Input: part model. Units: mm. Frame: model coordinates. Face numbers are marked on the shaded views. A direction names the side the tool comes from. Round coordinates to 2 decimals unless told otherwise and drop trailing zeros. Loops run counter-clockwise (first coordinate to the right, second up) from the corner with the lowest first, then second, coordinate; pieces in that order, holes last.
(1) Cut plane A-A, the plane y = 19. Output: boundary loops of the cut face in (x, z).
(2) First-contact query: pin 1 Ø2 at (y, z) = (48.5, 7.5) entering from +X; pin 2 Ø1.2 at (x, z) = (141, 14) entering from -Y; pin 3 Ø4.5 at (x, y) = (135.5, 22.5) entering from +Z; pin 4 Ø3 at (x, z) = (141.5, 14) entering from -Y. Flat tips, straight axial feed; report the tip coordinate or a pass-through.
(3) Cut plane B-B, the plane x = 141.5. Give the number of separate pieces and of enclosed holes in the cut face, and give its area (3 significant figures).
(4) Draft query along Y for the marked faces 5, 6 and 7. Return one class per face: released by +Y, released by -Y, zero draft, split by the parting line, or undercut.
(5) Cut plane C-C, the plane y = 31. Output: boundary loops of the cut face in (x, z).
(6) Cut plane D-D, the plane x = 147.5. Output: boundary loops of the cut face in (y, z).
(7) Line query: line 1 (Y direction, x = 133, z = 14); line 2 (Z direction, x = 141.5, y = 65); line 3 (Y direction, x = 136.75, z = 14). Output: solid intervals per line, ascending.
(8) Access query for the marked faces 1, 2, 3 and 4. Directions: +Z, -Z, +X, -X, +Y, -Y. A direction counts if a zero-diameter tool reaches every point of the face in a straight line with its end or side. Return the directions, or none.
from build123d import *

# Parameters (mm, degrees)
CYLINDER357_R     = 3
CYLINDER357_DEPTH = 17
CYLINDER356_R     = 3
CYLINDER356_DEPTH = 17
BOX221_W          = 5
BOX221_H          = 8
BOX221_DEPTH      = 10
FILLET089_R       = 2
BOX222_W          = 5
BOX222_H          = 60
BOX222_DEPTH      = 10
BOX217_W          = 1
BOX217_H          = 32
BOX217_DEPTH      = 22
CYLINDER297_R     = 1.6
CYLINDER297_DEPTH = 16
CYLINDER296_R     = 1.6
CYLINDER296_DEPTH = 16
CYLINDER295_R     = 1.25
CYLINDER295_DEPTH = 10
CYLINDER293_R     = 1.25
CYLINDER293_DEPTH = 10
CYLINDER294_R     = 1.25
CYLINDER294_DEPTH = 10
CYLINDER292_R     = 1.25
CYLINDER292_DEPTH = 10
CYLINDER291_R     = 3.5
CYLINDER291_DEPTH = 4
CYLINDER289_R     = 6.5
CYLINDER289_DEPTH = 4
BOX218_W          = 15
BOX218_H          = 16
BOX218_DEPTH      = 5.5
CYLINDER290_R     = 8
CYLINDER290_DEPTH = 10
BOX216_W          = 10
BOX216_H          = 80
BOX216_DEPTH      = 10
BOX219_W          = 5
BOX219_H          = 80
BOX219_DEPTH      = 10
FILLET090_R       = 2
BOX220_W          = 5
BOX220_H          = 8
BOX220_DEPTH      = 10
FILLET088_R       = 2
CHAMFER031_SIZE   = 5.49
CHAMFER032_SIZE   = 3
FILLET110_R       = 4.99


with BuildPart() as cylinder357:
    # Cylinder357 → Cylinder357 (new body)
    with BuildSketch(Plane(origin=(129, 57, 19), x_dir=(0, 0, -1), z_dir=(1, 0, 0))):
        Circle(CYLINDER357_R)
    extrude(amount=CYLINDER357_DEPTH)


with BuildPart() as fusion302:
    # Cylinder356 → Cylinder356 (new body)
    with BuildSketch(Plane(origin=(129, 5, 19), x_dir=(0, 0, -1), z_dir=(1, 0, 0))):
        Circle(CYLINDER356_R)
    extrude(amount=CYLINDER356_DEPTH)

    # Fusion302: union Cylinder357
    add(cylinder357.part)


with BuildPart() as fillet089:
    # Box221 → Box221 (new body)
    with BuildSketch(Plane(origin=(90, 53, 9), x_dir=(1, 0, 0), z_dir=(0, 0, 1))):
        with Locations((2.5, 4)):
            Rectangle(BOX221_W, BOX221_H)
    extrude(amount=BOX221_DEPTH)

    # Fillet089
    fillet089_edges = [fillet089.edges().sort_by_distance(p)[0] for p in [
        (92.5, 61, 19),
    ]]
    fillet(fillet089_edges, radius=FILLET089_R)


with BuildPart() as fillet089_1:
    # Fillet089 placement: moved
    add(fillet089.part.moved(Location((0, 10, 0))))


with BuildPart() as cube302:
    # Box222 → Box222 (new body)
    with BuildSketch(Plane(origin=(75, 1, -1), x_dir=(1, 0, 0), z_dir=(0, 0, 1))):
        with Locations((2.5, 30)):
            Rectangle(BOX222_W, BOX222_H)
    extrude(amount=BOX222_DEPTH)


with BuildPart() as cube297:
    # Box217 → Box217 (new body)
    with BuildSketch(Plane(origin=(89, 15, 2), x_dir=(1, 0, 0), z_dir=(0, 0, 1))):
        with Locations((0.5, 16)):
            Rectangle(BOX217_W, BOX217_H)
    extrude(amount=BOX217_DEPTH)


with BuildPart() as cylinder297:
    # Cylinder297 → Cylinder297 (new body)
    with BuildSketch(Plane(origin=(80, 43, 14), x_dir=(0, 0, -1), z_dir=(1, 0, 0))):
        Circle(CYLINDER297_R)
    extrude(amount=CYLINDER297_DEPTH)


with BuildPart() as fusion262:
    # Cylinder296 → Cylinder296 (new body)
    with BuildSketch(Plane(origin=(80, 19, 14), x_dir=(0, 0, -1), z_dir=(1, 0, 0))):
        Circle(CYLINDER296_R)
    extrude(amount=CYLINDER296_DEPTH)

    # Fusion262: union Cylinder297
    add(cylinder297.part)


with BuildPart() as fusion262_1:
    # Fusion262 placement: moved
    add(fusion262.part.moved(Location((-6, 0, 0))))


with BuildPart() as cylinder295:
    # Cylinder295 → Cylinder295 (new body)
    with BuildSketch(Plane(origin=(87.5, 71, 14), x_dir=(1, 0, 0), z_dir=(0, -1, 0))):
        Circle(CYLINDER295_R)
    extrude(amount=CYLINDER295_DEPTH)


with BuildPart() as fusion260:
    # Cylinder293 → Cylinder293 (new body)
    with BuildSketch(Plane(origin=(87.5, 1, 14), x_dir=(1, 0, 0), z_dir=(0, -1, 0))):
        Circle(CYLINDER293_R)
    extrude(amount=CYLINDER293_DEPTH)

    # Fusion260: union Cylinder295
    add(cylinder295.part)


with BuildPart() as cylinder294:
    # Cylinder294 → Cylinder294 (new body)
    with BuildSketch(Plane(origin=(82.5, 71, 14), x_dir=(1, 0, 0), z_dir=(0, -1, 0))):
        Circle(CYLINDER294_R)
    extrude(amount=CYLINDER294_DEPTH)


with BuildPart() as fusion261:
    # Cylinder292 → Cylinder292 (new body)
    with BuildSketch(Plane(origin=(82.5, 1, 14), x_dir=(1, 0, 0), z_dir=(0, -1, 0))):
        Circle(CYLINDER292_R)
    extrude(amount=CYLINDER292_DEPTH)

    # Fusion259: union Cylinder294
    add(cylinder294.part)

    # Fusion261: union Fusion260
    add(fusion260.part)


with BuildPart() as cylinder291:
    # Cylinder291 → Cylinder291 (new body)
    with BuildSketch(Plane(origin=(89.5, 31, 10), x_dir=(0, 0, -1), z_dir=(1, 0, 0))):
        Circle(CYLINDER291_R)
    extrude(amount=CYLINDER291_DEPTH)


with BuildPart() as fusion257:
    # Cylinder289 → Cylinder289 (new body)
    with BuildSketch(Plane(origin=(90, 31, 10), x_dir=(0, 0, -1), z_dir=(1, 0, 0))):
        Circle(CYLINDER289_R)
    extrude(amount=CYLINDER289_DEPTH)

    # Fusion257: union Cylinder291
    add(cylinder291.part)


with BuildPart() as fusion257_1:
    # Fusion257 placement: moved
    add(fusion257.part.moved(Location((-4, 0, 2))))


with BuildPart() as cube298:
    # Box218 → Box218 (new body)
    with BuildSketch(Plane(origin=(75, 23, 3.5), x_dir=(1, 0, 0), z_dir=(0, 0, 1))):
        with Locations((7.5, 8)):
            Rectangle(BOX218_W, BOX218_H)
    extrude(amount=BOX218_DEPTH)


with BuildPart() as cylinder290:
    # Cylinder290 → Cylinder290 (new body)
    with BuildSketch(Plane(origin=(80, 31, 11.5), x_dir=(0, 0, -1), z_dir=(1, 0, 0))):
        Circle(CYLINDER290_R)
    extrude(amount=CYLINDER290_DEPTH)


with BuildPart() as fusion258:
    # Box216 → Box216 (new body)
    with BuildSketch(Plane(origin=(80, -9, 9), x_dir=(1, 0, 0), z_dir=(0, 0, 1))):
        with Locations((5, 40)):
            Rectangle(BOX216_W, BOX216_H)
    extrude(amount=BOX216_DEPTH)

    # Fusion258: union Cylinder290
    add(cylinder290.part)


with BuildPart() as fillet090:
    # Box219 → Box219 (new body)
    with BuildSketch(Plane(origin=(75, -9, 9), x_dir=(1, 0, 0), z_dir=(0, 0, 1))):
        with Locations((2.5, 40)):
            Rectangle(BOX219_W, BOX219_H)
    extrude(amount=BOX219_DEPTH)

    # Fusion263: union Cube298, Fusion258
    add(cube298.part)
    add(fusion258.part)

    # Cut226: cut Fusion257
    add(fusion257_1.part, mode=Mode.SUBTRACT)

    # Cut227: cut Fusion261
    add(fusion261.part, mode=Mode.SUBTRACT)

    # Cut228: cut Fusion262
    add(fusion262_1.part, mode=Mode.SUBTRACT)

    # Cut229: cut Cube297
    add(cube297.part, mode=Mode.SUBTRACT)

    # Cut230: cut Cube302
    add(cube302.part, mode=Mode.SUBTRACT)

    # Fillet090
    fillet090_edges = [fillet090.edges().sort_by_distance(p)[0] for p in [
        (82.5, -9, 19),
        (82.5, 71, 19),
    ]]
    fillet(fillet090_edges, radius=FILLET090_R)


with BuildPart() as front_threaded_bar_support_wide:
    # Box220 → Box220 (new body)
    with BuildSketch(Plane(origin=(90, 1, 9), x_dir=(1, 0, 0), z_dir=(0, 0, 1))):
        with Locations((2.5, 4)):
            Rectangle(BOX220_W, BOX220_H)
    extrude(amount=BOX220_DEPTH)

    # Fillet088
    fillet088_edges = [front_threaded_bar_support_wide.edges().sort_by_distance(p)[0] for p in [
        (92.5, 1, 19),
    ]]
    fillet(fillet088_edges, radius=FILLET088_R)


with BuildPart() as front_threaded_bar_support_wide_1:
    # Fillet088 placement: moved
    add(front_threaded_bar_support_wide.part.moved(Location((0, -10, 0))))

    # Fusion264: union Fillet089, Fillet090
    add(fillet089_1.part)
    add(fillet090.part)


with BuildPart() as front_threaded_bar_support_wide_2:
    # Fusion264 placement: moved
    add(front_threaded_bar_support_wide_1.part.moved(Location((54, 0, 0))))

    # Cut305: cut Fusion302
    add(fusion302.part, mode=Mode.SUBTRACT)

    # Chamfer031
    chamfer031_edges = [front_threaded_bar_support_wide_2.edges().sort_by_distance(p)[0] for p in [
        (138.5, 39, 9),
        (138.5, 23, 9),
    ]]
    chamfer(chamfer031_edges, length=CHAMFER031_SIZE)

    # Chamfer032
    chamfer032_edges = [front_threaded_bar_support_wide_2.edges().sort_by_distance(p)[0] for p in [
        (134, 31, 3.5),
    ]]
    chamfer(chamfer032_edges, length=CHAMFER032_SIZE)

    # Fillet110
    fillet110_edges = [front_threaded_bar_support_wide_2.edges().sort_by_distance(p)[0] for p in [
        (144, 63, 14),
        (144, -1, 14),
    ]]
    fillet(fillet110_edges, radius=FILLET110_R)


solid = front_threaded_bar_support_wide_2.part
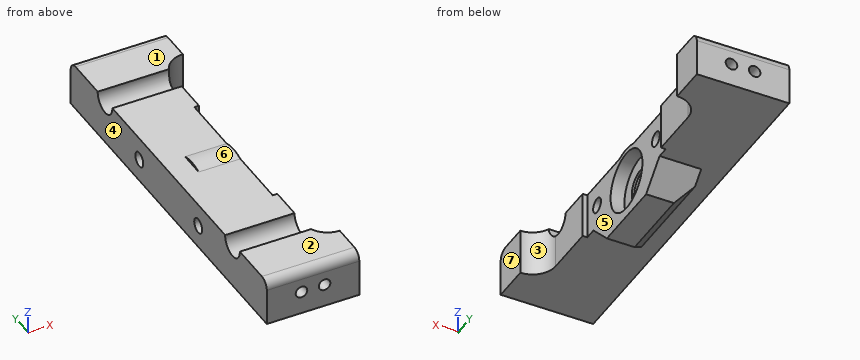
Reported:
1. outline: (129, 9) - (134, 9) - (134, 7.51) - (143, 7.51) - (143, 12.4) - (129, 12.4) - close; (129, 15.6) - (143, 15.6) - (143, 19) - (129, 19) - close
2. pin 1: passes through
2. pin 2: stops at y = 1
2. pin 3: stops at z = 19
2. pin 4: stops at y = -9
3. separate pieces: 1
3. enclosed holes: 3
3. area: 691 mm2
4. face 5: undercut
4. face 6: split by the parting line
4. face 7: zero draft
5. outline: (129, 9) - (134, 9) - (134, 6.5) - (137, 3.5) - (143, 3.5) - (143, 5.5) - (140, 5.5) - (140, 8.5) - (139.5, 8.5) - (139.5, 15.5) - (140, 15.5) - (140, 18.5) - (143, 18.5) - (143, 19.5) - (134, 19.5) - (134, 19) - (129, 19) - close
6. outline: (-9, 9) - (-0.77, 9) - (-0.77, 19) - (-7, 19) arc R2 ccw to (-9, 17) - close; (62.77, 9) - (71, 9) - (71, 17) arc R2 ccw to (69, 19) - (62.77, 19) - close
7. line 1: y = -9 to 17.4, 20.6 to 41.4, 44.6 to 71
7. line 2: z = 9 to 12.75, 15.25 to 19
7. line 3: y = 1 to 17.4, 20.6 to 41.4, 44.6 to 61
8. face 1: +Z, +X, -X, +Y
8. face 2: +Z, +X, -X, -Y
8. face 3: +Z, -Z, +X
8. face 4: +Z, -Z, -X, +Y, -Y
